Part model, mm, in its own coordinate system. Face numbers are marked on the shaded views. A direction names the side the tool comes from. Round coordinates to 2 decimals unless told otherwise and drop trailing zeros. Write each loop counter-clockwise with the first axis right and the second up, starting at its lowest first coordinate (ties: lowest second). Pieces come first, ordered by that corner, then holes. Notation, with made-up numbers: (57.25, -5) -> (108.25, -5) arc R5 ccw to (108.25, 4) -> close; hole circle Ø2 at (83.25, 54). An arc over 180 degrees is marked (long way). Return JSON: item names as keys, results as strings. Group by question number.
(1) Drill centre lines: L1, parallel to X at y = 0.25, z = 82.5; L2, parallel to Z at x = 5.75, y = -2.25; L3, parallel to Z at x = -0.25, y = -1.5. Where is each one in solid material? Low to high. Write a range as from..to.
(2) Tool access for the marked faces 1 and 2: list every direction of +Z, -Z, +X, -X, +Y, -Y with a clear straight run to the whole face (end or side of a thin tool).
(3) Drop flat-ended pins along their axis: pin 1 Ø2 at (y, z) = (-6, 41.5) entering from -X; pin 2 Ø6 at (y, z) = (-7, 84.5) entering from -X; pin 3 Ø1 at (x, y) = (-9.5, 3) entering from +Z. Give the stop position or say it passes through.
(4) Saw through at B-B (z = 51). List the corners of the cut face in (x, y), plus the area to 3 significant figures.
(5) Saw through at A-A (z = 7). List the corners of the cut face in (x, y).
from build123d import *

# Parameters (mm, degrees)
F0_R     = 13
F1_DEPTH = 10
F2_R     = 6.002605
F3_DEPTH = 90
F4_R     = 5
F5_R     = 5


with BuildPart() as f1:
    # F0 (on Top) → F1 (new body)
    with BuildSketch(Plane.XY):
        Circle(F0_R)
    extrude(amount=F1_DEPTH)

    # F2 (on face) → F3 (join)
    with BuildSketch(Plane.XY.offset(10)):
        Circle(F2_R)
    extrude(amount=F3_DEPTH)

    # F4
    f4_edges = [f1.edges().sort_by_distance(p)[0] for p in [
        (-13, 0, 0),
    ]]
    fillet(f4_edges, radius=F4_R)

    # F5
    f5_edges = [f1.edges().sort_by_distance(p)[0] for p in [
        (-6.002605, 0, 100),
    ]]
    fillet(f5_edges, radius=F5_R)


solid = f1.part
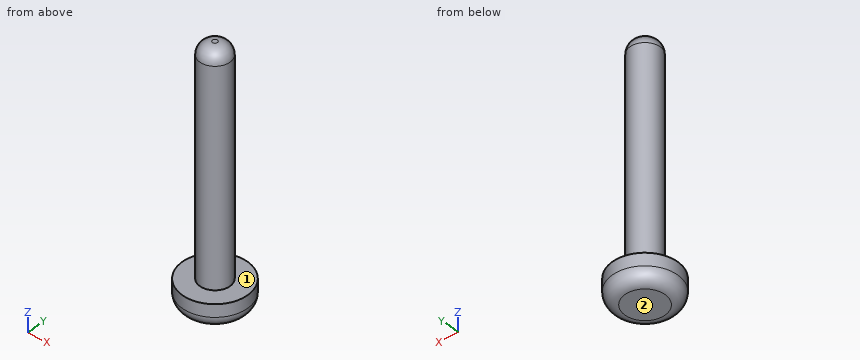
Computed values:
{
 "1": {"L1": "-6..6", "L2": "0..10", "L3": "0..99.97"},
 "2": {"face 1": "+Z", "face 2": "-Z, +X, -X, +Y, -Y"},
 "3": {"pin 1": "x = -3.32", "pin 2": "x = -4.48", "pin 3": "z = 10"},
 "4": {"outline": "circle Ø12.01 at (0, 0)", "area": "113 mm2"},
 "5": {"outline": "circle Ø26 at (0, 0)"}
}
